Geometry check sheet. Reference: the model listing, model coordinates, mm. Round coordinates to 2 decimals unless told otherwise and drop trailing zeros. Write each loop counter-clockwise with the first axis right and the second up, starting at its lowest first coordinate (ties: lowest second). Pieces come first, ordered by that corner, then holes. Notation, with made-up numbers: M -18,10 L 6,10 A24 ccw 6,42 Z; hole C -1,48 d4. An arc over 180 degrees is marked long. One line per item, written item: value. Start each with the question number.
1. Section check C-C (z = 9). Record the boundary of the cut face in (x, y).
2. Depth check by flat-ended pin: P1, Ø2, axis at y = -5, z = 1, coming from the +X side; P2, Ø6, axis at y = 1, z = 5.5, coming from the -X side. Enter the tip coordinate at first touch or a pass-through.
3. Section check B-B (x = 19.5). Record the boundary of the cut face in (y, z), and give its area (3 significant figures).
4. Section check A-A (y = 4.25). Record the boundary of the cut face in (x, z).
5. Section check D-D (x = -3). Record the boundary of the cut face in (y, z).
6. Scan lines: probe 1 along Y at (x, z) = (17, 4.5); probe 2 along Y at (x, z) = (18.25, 1); probe 3 along X at (y, z) = (5.75, 9.5). Record each from-to range of solid material in increasing order. Write a range as [from, to].
7. Release check for a two-part mould opening along X. For faces 1 (the cylindrical face through (21.252, -9.437, 5.07)), 2 (the cylindrical face through (-3.483, 6.783, 4.93)), 3 (the flat face through (7, -2, 0)) record: pulls with the +X half, pulls with the -X half, needs draft (parallel to the pull), parting line crosses it, or undercut.
Autodesk Inventor part; units mm, degrees
ref_plane "YZ Plane" through (0, 0, 0) normal (1, 0, 0) x (0, 1, 0)
ref_plane "XZ Plane" through (0, 0, 0) normal (0, 1, 0) x (-1, 0, 0)
ref_plane "XY Plane" through (0, 0, 0) normal (0, 0, 1) x (1, 0, 0)
sketch "Sketch1" plane through (0, 0, 0) normal (0, 0, 1) x (1, 0, 0)
  line L0 (-13.9136, 8.9772) -> (28.0864, 8.9772)
  line L1 (28.0864, 8.9772) -> (28.0864, -13.0228)
  line L2 (28.0864, -13.0228) -> (-13.9136, -13.0228)
  line L3 (-13.9136, -13.0228) -> (-13.9136, 8.9772)
  point P0 (0, 0)
  dimension "d0" = 42
  dimension "d1" = 22
extrude "Extrusion1" add sketch "Sketch1" along normal blind 10
sketch "Sketch2" plane through (0, 0, 10) normal (0, 0, 1) x (1, 0, 0)
  line L0 (-13.9136, -13.0228) -> (28.0864, -13.0228)
  arc A0 (-3.4134, -5.6894) -> (-3.4136, -13.0228) centre (-3.4136, -9.3561) ccw
  arc A1 (-3.4134, -5.6894) -> (-3.4134, 1.6439) centre (-3.4133, -2.0228) ccw
  arc A2 (17.5864, -13.0228) -> (17.5862, -5.6894) centre (17.5864, -9.3561) ccw
  arc A3 (17.5862, 1.6439) -> (17.5862, -5.6894) centre (17.586, -2.0228) ccw
  line L1 (-3.4136, -13.0228) -> (17.5864, -13.0228)
  line L2 (-3.4135, 8.9772) -> (17.5865, 8.9772)
  line L3 (28.0864, 8.9772) -> (-13.9136, 8.9772)
  line L4 (-3.4133, -2.0228) -> (-3.4136, -9.3561) construction
  line L5 (17.5864, -9.3561) -> (17.586, -2.0228) construction
  arc A4 (-3.4135, 8.9772) -> (-3.4134, 1.6439) centre (-3.4136, 5.3106) ccw
  arc A5 (17.5862, 1.6439) -> (17.5865, 8.9772) centre (17.5864, 5.3106) ccw
  line L6 (-3.4133, -2.0228) -> (-13.9136, -2.0228) construction
  line L7 (17.586, -2.0228) -> (28.0864, -2.0228) construction
  line L8 (28.0864, -13.0228) -> (28.0864, 8.9772) construction
  line L9 (-13.9136, 8.9772) -> (-13.9136, -13.0228)
  line L10 (-7.0803, -9.356) -> (-13.9136, -9.356) construction
  line L11 (21.2531, -9.356) -> (28.0864, -9.356) construction
  line L12 (-13.9136, -13.0228) -> (28.0864, -13.0228)
  line L13 (28.0864, -13.0228) -> (28.0864, 8.9772)
  line L14 (28.0864, 8.9772) -> (-13.9136, 8.9772)
  line L15 (-13.9136, 8.9772) -> (-13.9136, -13.0228)
  line L16 (-7.0803, 5.3105) -> (-13.9136, 5.3105) construction
  line L17 (21.2531, 5.3105) -> (28.0864, 5.3105) construction
  point P0 (0, 0)
  point P1 (17.8152, 8.9772)
  point P2 (-3.4136, 8.9772)
  point P3 (-3.4136, 8.9772)
  dimension "d4" = 21
  dimension "d5" = 22
  dimension "d17" = 21
extrude "Extrusion2" cut sketch "Sketch2" against normal blind 10 contours L9 L3 A4 A1 A0 L0 | A2 A3 A5 L3 L13 L0
sketch "Sketch3" plane through (0, 0, 10) normal (0, 0, 1) x (1, 0, 0)
  arc A0 (-3.4134, -5.6894) -> (-3.4134, 1.6439) centre (-3.4133, -2.0228) ccw construction
  line L0 (-7.2207, -5.6893) -> (3.1864, -5.6897) construction
  line L1 (20.3968, -5.6893) -> (9.686, -5.6898) construction
  arc A1 (-3.4134, -5.6894) -> (-3.4136, -13.0228) centre (-3.4136, -9.3561) ccw construction
  arc A2 (-3.4134, -5.6894) -> (-3.4134, 1.6439) centre (-3.4133, -2.0228) ccw construction
  arc A3 (17.5864, -13.0228) -> (17.5862, -5.6894) centre (17.5864, -9.3561) ccw construction
  arc A4 (17.5862, 1.6439) -> (17.5862, -5.6894) centre (17.586, -2.0228) ccw construction
  line L2 (-3.4137, -11.3763) -> (-3.4129, 5.1845) construction
  line L3 (17.5866, -13.0364) -> (17.5857, 5.1238) construction
  arc A5 (17.5862, 1.6439) -> (17.5862, -5.6894) centre (17.586, -2.0228) ccw construction
  point P0 (0, 0)
hole "Hole1" at (17.5857, 5.1238, 10) direction (0, 0, -1) diameter 3 end through all
hole "Hole2" at (-3.4129, 5.1845, 10) direction (0, 0, -1) diameter 3.2 end through all
properties part number "Zipperteethv7"
Result sheet:
1. outline: M -3.41,-13.02 L 17.59,-13.02 A3.67 ccw 17.59,-5.69 A3.67 cw 17.59,1.64 A3.67 ccw 17.59,8.98 L -3.41,8.98 A3.67 ccw -3.41,1.64 A3.67 cw -3.41,-5.69 A3.67 ccw Z; hole C -3.41,5.18 d3.2; hole C 17.59,5.12 d3
2. P1: stops at x = 19.06
2. P2: stops at x = -6.84
3. outline: M -12.48,0 L -6.23,0 L -6.23,10 L -12.48,10 Z; M 2.18,0 L 8.44,0 L 8.44,10 L 2.18,10 Z
3. area: 125 mm2
4. outline: M -6.92,0 L -4.71,0 L -4.71,10 L -6.92,10 Z; M -2.11,0 L 16.37,0 L 16.37,10 L -2.11,10 Z; M 18.8,0 L 21.1,0 L 21.1,10 L 18.8,10 Z
5. outline: M -13.02,0 L -5.67,0 L -5.67,10 L -13.02,10 Z; M 1.62,0 L 3.64,0 L 3.64,10 L 1.62,10 Z; M 6.73,0 L 8.98,0 L 8.98,10 L 6.73,10 Z
6. probe 1: y = [-13.02, -5.64], [1.6, 3.74], [6.5, 8.98]
6. probe 2: y = [-12.96, -5.75], [1.7, 3.78], [6.47, 8.92]
6. probe 3: x = [-7.05, -4.91], [-1.92, 16.22], [18.95, 21.23]
7. face 1: pulls with the +X half
7. face 2: undercut
7. face 3: needs draft
